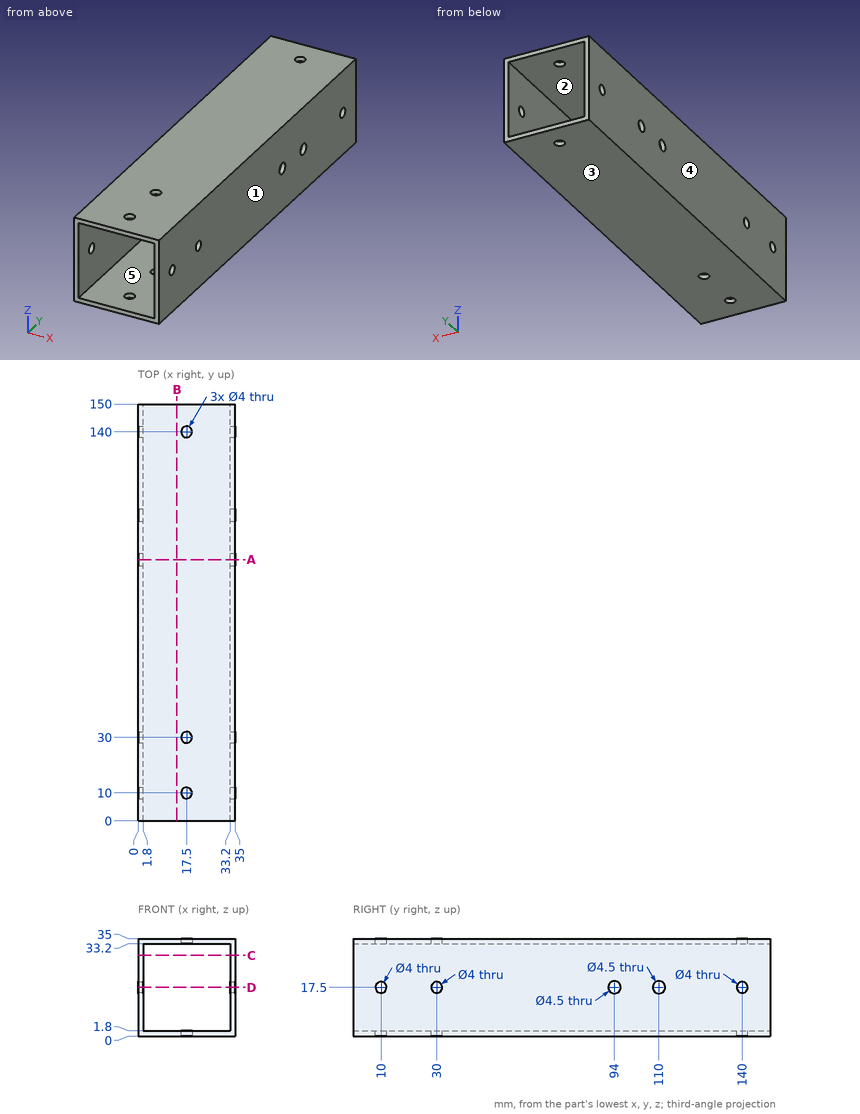
Source: three-view drawing plus pictorial views. Frame: mm from the lowest corner of the part. A direction names the side the tool comes from. Give positions to 0.01 mm unless a question says otherwise; leave off trailing zeros. Order: outer loops, then holes, each group sorted by start corner. A loop starts at its lowest first (then second) coordinate and runs counter-clockwise, first axis right, second up. Notation, with made-up numbers: (71, 65) -> (101, 65) arc R17 cw to (101, 95) -> close; hole circle Ø11 at (46.25, -16). An arc over 180 degrees is marked (long way). Put each result on its own line as item: value.
Q1. Section C-C, the plane z = 29. Return loops of the section in (x, y), then the cut area to 3 significant figures.
Here are the results:
outline: (0, 0) -> (1.8, 0) -> (1.8, 150) -> (0, 150) -> close; (33.2, 0) -> (35, 0) -> (35, 150) -> (33.2, 150) -> close
area: 540 mm^2
Q2. Section A-A, the plane y = 94. Return loops of the section in (x, z).
Here are the results:
outline: (0, 0) -> (35, 0) -> (35, 15.25) -> (33.2, 15.25) -> (33.2, 1.8) -> (1.8, 1.8) -> (1.8, 15.25) -> (0, 15.25) -> close; (0, 19.75) -> (1.8, 19.75) -> (1.8, 33.2) -> (33.2, 33.2) -> (33.2, 19.75) -> (35, 19.75) -> (35, 35) -> (0, 35) -> close
Q3. Section B-B, the plane x = 14. Return loops of the section in (y, z), then the cut area to 3 significant figures.
Here are the results:
outline: (0, 0) -> (150, 0) -> (150, 1.8) -> (0, 1.8) -> close; (0, 33.2) -> (150, 33.2) -> (150, 35) -> (0, 35) -> close
area: 540 mm^2
Q4. Reachability of the marked faces 4 and 5 from +Z, -Z, +X, -X, +Y, -Y: full face, straight path, thin tool, end or side. Return the list, or none.
Here are the results:
face 4: +Z, -Z, -X, +Y, -Y
face 5: +Y, -Y
Q5. Material intervals for L1, parallel to Y at x = 34.35, z = 17.5; L2, parallel to Y at x = 17.5, z = 33.9; L3, parallel to Z at x = 9, y = 87, sorted ascending.
Here are the results:
L1: y = 0 to 8, 12 to 28, 32 to 91.75, 96.25 to 107.75, 112.25 to 138, 142 to 150
L2: y = 0 to 8, 12 to 28, 32 to 138, 142 to 150
L3: z = 0 to 1.8, 33.2 to 35
Q6. Section D-D, the plane z = 17.5. Count the separate pieces of the cut face and the enclosed holes in it, then the cut area to 3 significant figures.
Here are the results:
separate pieces: 12
enclosed holes: 0
area: 464 mm^2
Q7. Pin query (flat end, axial travel): pin 1 (3.5 mm diameter, centred on y = 10, z = 17.5, fed in from -X). Return the tip coordinate at first contact, or that it passes through.
Here are the results:
pin 1: passes through
Q8. Draft query along Z for the marked faces 1, 2 and 3. Return one class per face: released by +Z, released by -Z, zero draft, split by the parting line, or undercut.
Here are the results:
face 1: zero draft
face 2: undercut
face 3: released by -Z
